```python
from build123d import *

# Parameters (mm, degrees)
F0_R     = 25
F0_R_2   = 4.75
F1_DEPTH = 5
F2_R     = 10


with BuildPart() as f1:
    # F0 (on Top) → F1 (new body)
    with BuildSketch(Plane.XY):
        with BuildLine():
            ThreePointArc((130.202041, 5), (79.383877, 9), (28.565714, 5))
            ThreePointArc((28.565714, 5), (-29, 0), (28.565714, -5))
            ThreePointArc((28.565714, -5), (79.383877, -9), (130.202041, -5))
            ThreePointArc((130.202041, -5), (151, 0), (130.202041, 5))
        make_face()
        Circle(F0_R, mode=Mode.SUBTRACT)
        with Locations((140, 0)):
            Circle(F0_R_2, mode=Mode.SUBTRACT)
    extrude(amount=F1_DEPTH)

    # F2
    f2_edges = [f1.edges().sort_by_distance(p)[0] for p in [
        (28.565714, -5, 2.5),
        (28.565714, 5, 2.5),
        (130.202041, 5, 2.5),
        (130.202041, -5, 2.5),
    ]]
    fillet(f2_edges, radius=F2_R)


solid = f1.part
```
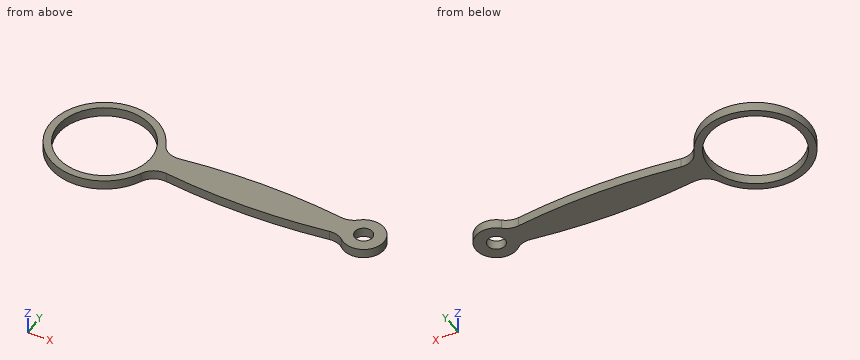
Geometry: final body of the model. Coordinates: model frame, mm. Round coordinates to 2 decimals unless told otherwise and drop trailing zeros. Order: outer loops, then holes, each group sorted by start corner. A loop starts at its lowest first (then second) coordinate and runs counter-clockwise, first axis right, second up. Notation, with made-up numbers: (61, -30) -> (87, -30) arc R31 cw to (87, -6) -> close; hole circle Ø2 at (-16.75, 65). An arc over 180 degrees is marked (long way). Use one line per item in the form item = value.
(1) Section A-A on x = 0. Return loops of the section in (y, z), and give its area (3 significant figures).
Results list:
outline = (-29, 0) -> (-25, 0) -> (-25, 5) -> (-29, 5) -> close; (25, 0) -> (29, 0) -> (29, 5) -> (25, 5) -> close
area = 40.0 mm^2
(2) First-contact query: pin 1 Ø2 at (y, z) = (17.5, 1) entering from +X; pin 2 Ø1 at (y, z) = (-14.5, 0.5) entering from -X. Flat tips, straight axial feed; report the tip coordinate or a pass-through.
Results list:
pin_1 = 23.85
pin_2 = -25.4
(3) Section D-D on z = 2.1. Count the separate pieces of the cut face and the enclosed holes in it, and give its area (3 significant figures).
Results list:
separate_pieces = 1
enclosed_holes = 2
area = 2,570 mm^2
(4) Ray query, probe 1 along Y at (x, z) = (0, 3.8); probe 2 along Y at (x, z) = (140, 2.9); probe 3 along X at (y, z) = (-9.5, 3.4). Return the intervals inside material, ascending. Write a range as [from, to].
Results list:
probe_1 = [-29, -25], [25, 29]
probe_2 = [-11, -4.75], [4.75, 11]
probe_3 = [-27.4, -23.12], [23.12, 28.01], [134.45, 145.55]
(5) Section C-C on y = -21.5. Return loops of the section in (x, z), and give its area (3 significant figures).
Results list:
outline = (-19.46, 0) -> (-12.76, 0) -> (-12.76, 5) -> (-19.46, 5) -> close; (12.76, 0) -> (19.46, 0) -> (19.46, 5) -> (12.76, 5) -> close
area = 67.0 mm^2
(6) Section B-B on y = 0. Return loops of the section in (x, z).
Results list:
outline = (-29, 0) -> (-25, 0) -> (-25, 5) -> (-29, 5) -> close; (25, 0) -> (135.25, 0) -> (135.25, 5) -> (25, 5) -> close; (144.75, 0) -> (151, 0) -> (151, 5) -> (144.75, 5) -> close
